The listing builds one solid part. Answer for the finished solid, in the listing's coordinates (mm). Give positions to 0.01 mm unless a question says otherwise; leave off trailing zeros. Write each loop counter-clockwise with the first axis right and the second up, starting at its lowest first coordinate (ties: lowest second). Pieces come first, ordered by that corner, then holes. Notation, with made-up numbers: M 87,74 L 106,74 A17 cw 106,83 Z; hole C 50.5,47.5 d4. An arc over 180 degrees is marked long. Return JSON: item names as keys, results as strings.
Autodesk Inventor part; units mm, degrees
ref_plane "YZ Plane" through (0, 0, 0) normal (1, 0, 0) x (0, 1, 0)
ref_plane "XZ Plane" through (0, 0, 0) normal (0, 1, 0) x (-1, 0, 0)
ref_plane "XY Plane" through (0, 0, 0) normal (0, 0, 1) x (1, 0, 0)
sketch "Sketch3" plane through (0, 0, 0) normal (1, 0, 0) x (0, 1, 0)
  circle A0 centre (0, 0) radius 14
  line L0 (-23, -102.8316) -> (23, -102.8316)
  line L1 (23, -102.8316) -> (23, 102.8316)
  line L2 (23, 102.8316) -> (-23, 102.8316)
  line L3 (-23, 102.8316) -> (-23, -102.8316)
  line L4 (-23, -102.8316) -> (23, 102.8316) construction
  line L5 (23, -102.8316) -> (-23, 102.8316) construction
  circle A1 centre (17, -15) radius 2.5
  circle A2 centre (-17, 12) radius 2.5
  circle A3 centre (17, -15) radius 6
  circle A4 centre (-17, 12) radius 6
  line L6 (-22.0787, 8.8052) -> (-11.8503, -7.4546)
  line L7 (-4.9626, -13.0909) -> (14.8732, -20.6104)
  line L8 (12.3712, 6.554) -> (22.3019, -12.1912)
  line L9 (3.0558, 13.6624) -> (-15.6904, 17.8553)
  dimension "d11" = 28
  dimension "d12" = 46
  dimension "d13" = 5
  dimension "d14" = 6
  dimension "d15" = 6
  dimension "d16" = 12
  dimension "d17" = 15
extrude "Extrusion3" add sketch "Sketch3" along normal blind 5 contours A0 | A0 L8 A3 L7 | A0 L6 A4 L9 | A3 | A4
properties part number "frame_center"
Item 1: A cutting plane is placed at D-D, the plane z = 3. Write down the section's boundary in (x, y), plus the area to 3 significant figures.
Geometry results:
{"outline": "M 0,-18.43 L 5,-18.43 L 5,14.25 L 0,14.25 Z", "area": "163 mm2"}
Item 2: Find the intervals of material crossed by line 1 (Z direction, x = 3.35, y = 18); line 2 (Z direction, x = 4.7, y = -16); line 3 (Y direction, x = 4.75, z = 10.5), in increasing order.
Geometry results:
{"line 1": "z = -20.92 to -17.29, -12.71 to -4.07", "line 2": "z = -0.86 to 9.71, 14.29 to 17.92", "line 3": "y = -22.81 to -19, -15 to 9.26"}
Item 3: Determine the mould class of faces 1 (the cylindrical face through (2.5, 8.4, 11.2)), 2 (the cylindrical face through (2.46, -8.82, -10.87)), 3 (the cylindrical face through (2.5, 14.5, -15.1)) for opening direction Y: +Y half, -Y half, draft (parallel to the pull), parting line (faces both ways), or undercut.
Geometry results:
{"face 1": "+Y half", "face 2": "-Y half", "face 3": "undercut"}
Item 4: Given pin 1 Ø2 at (x, z) = (3, 12) entering from +Y; pin 2 Ø1.5 at (x, z) = (2.5, 7.5) entering from +Y; pin 3 Ø3 at (x, z) = (2, 8.5) entering from -Y, each flat-ended and moving along its own axis, determine where each tip first touches the part or whether it passes through.
Geometry results:
{"pin 1": "stops at y = 8.66", "pin 2": "stops at y = 12.27", "pin 3": "stops at y = -22.66"}
Item 5: A cutting plane is placed at B-B, the plane z = 12. Write down the section's boundary in (x, y), plus the area to 3 significant figures.
Geometry results:
{"outline": "M 0,-23 L 5,-23 L 5,-19.5 L 0,-19.5 Z; M 0,-14.5 L 5,-14.5 L 5,7.21 L 0,7.21 Z", "area": "126 mm2"}
Item 6: A cutting plane is placed at C-C, the plane x = 3.2. Write down the section's boundary in (y, z).
Geometry results:
{"outline": "M -22.08,8.81 L -11.85,-7.45 A14 ccw -4.96,-13.09 L 14.87,-20.61 A6 ccw 22.3,-12.19 L 12.37,6.55 A14 ccw 3.06,13.66 L -15.69,17.86 A6 ccw Z; hole C -17,12 d5; hole C 17,-15 d5"}
Item 7: A cutting plane is placed at A-A, the plane y = 16. Write down the section's boundary in (x, z), plus the area to 3 significant figures.
Geometry results:
{"outline": "M 0,-20.92 L 5,-20.92 L 5,-17.29 L 0,-17.29 Z; M 0,-12.71 L 5,-12.71 L 5,-0.3 L 0,-0.3 Z", "area": "80.2 mm2"}
